Study the drawing (mm; zero at the part's minimum x, y, z) and answer. Round coordinates to 2 decimals unless told otherwise and drop trailing zeros. Loops run counter-clockwise (first coordinate to the right, second up) from the corner with the lowest first, then second, coordinate; pieces in that order, holes last. Notation, with made-up numbers: M 63.5,30 L 97.5,30 A21 cw 97.5,47 Z; hole C 70.25,-6 d5. An arc over 180 degrees is marked long. Write each question's results on one line, items separated by ' | '.
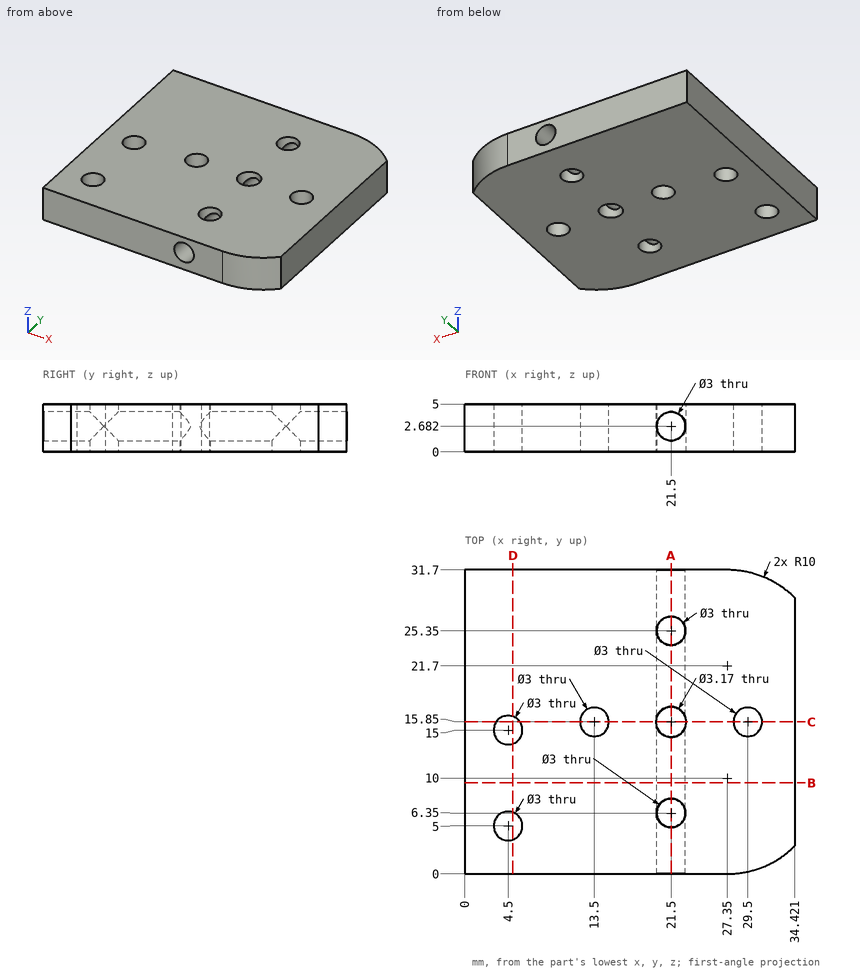
Item 1: A flat-ended cylindrical pin translates along its axis: pin 1 (4 mm diameter, centred on x = 4.5, y = 5, fed in from -Z). Find the tip coordinate at first contact, or state that the pin passes through.
Outcome:
pin 1: stops at z = 0
Item 2: The part is cut by section A-A (x = 21.5). State how many separate pieces and enclosed holes the cut face has.
Outcome:
separate pieces: 8 | enclosed holes: 0
Item 3: Straight lines are drawn through the part: line 1 (Y direction, x = 4.5, z = 3.7); line 2 (X direction, y = 8, z = 2.55); line 3 (Y direction, x = 13.5, z = 3.3). For each, find the intervals that lie inside material, in ascending order.
Outcome:
line 1: y = 0 to 3.5, 6.5 to 13.5, 16.5 to 31.7 | line 2: x = 0 to 20.01, 22.99 to 34.42 | line 3: y = 0 to 14.35, 17.35 to 31.7
Item 4: The part is cut by section D-D (x = 5). Determine the outline of the cut face in (y, z), plus the area to 3 significant figures.
Outcome:
outline: M 0,0 L 3.59,0 L 3.59,5 L 0,5 Z; M 6.41,0 L 13.59,0 L 13.59,5 L 6.41,5 Z; M 16.41,0 L 31.7,0 L 31.7,5 L 16.41,5 Z | area: 130 mm2
Item 5: The part is cut by section C-C (y = 15.85). Determine the outline of the cut face in (x, z) (3 decimals).
Outcome:
outline: M 0,0 L 3.264,0 L 3.264,5 L 0,5 Z; M 5.736,0 L 12,0 L 12,5 L 5.736,5 Z; M 15,0 L 19.915,0 L 19.915,5 L 15,5 Z; M 23.085,0 L 28,0 L 28,5 L 23.085,5 Z; M 31,0 L 34.421,0 L 34.421,5 L 31,5 Z
Item 6: The part is cut by section B-B (y = 9.5). Determine the outline of the cut face in (x, z).
Outcome:
outline: M 0,0 L 34.42,0 L 34.42,5 L 0,5 Z; hole C 21.5,2.68 d3
